from build123d import *

# Parameters (mm, degrees)
F0_W     = 60
F0_H     = 60
F1_DEPTH = 140
F2_R     = 16.4842483895
F2_R_2   = 17.1367396553
F2_R_3   = 16.9091823749
F3_DEPTH = 15
F4_DEPTH = 199
F5_DEPTH = 25
F6_DEPTH = 5


with BuildPart() as f1:
    # F0 (on Top) → F1 (new body)
    with BuildSketch(Plane.XY):
        with Locations((30, 30)):
            Rectangle(F0_W, F0_H)
    extrude(amount=F1_DEPTH)

    # F2 (on face) → F3 (join)
    with BuildSketch(Plane.XZ):
        with Locations((32.427366823, 110.1229637861)):
            Circle(F2_R)
        with Locations((32.427366823, 72.1417963505)):
            Circle(F2_R_2)
        with Locations((32.7129401267, 27.8780274093)):
            Circle(F2_R_3)
    extrude(amount=F3_DEPTH)

    # F4 (cut): a face of the model
    f4_faces = [f1.faces().sort_by_distance(p)[0] for p in [
        (32.427366823, -15, 72.1417963505),
    ]]
    extrude(f4_faces, amount=-F4_DEPTH, mode=Mode.SUBTRACT)

    # F5 (cut): a face of the model
    f5_faces = [f1.faces().sort_by_distance(p)[0] for p in [
        (32.427366823, -15, 110.1229637861),
    ]]
    extrude(f5_faces, amount=-F5_DEPTH, mode=Mode.SUBTRACT)

    # F6 (cut): a face of the model
    f6_faces = [f1.faces().sort_by_distance(p)[0] for p in [
        (32.7129401267, -15, 27.8780274093),
    ]]
    extrude(f6_faces, amount=-F6_DEPTH, mode=Mode.SUBTRACT)


solid = f1.part
Could you check a few things on this model? Use its own coordinates, in mm. A direction names the side the tool comes from. Round coordinates to 2 decimals unless told otherwise and drop trailing zeros. Order: outer loops, then holes, each group sorted by start corner. A loop starts at its lowest first (then second) coordinate and runs counter-clockwise, first axis right, second up.
(1) Imagine slicing it at D-D (z = 20). Write out the boundary of the cut face in (x, y).
Response values:
outline: (0, 0) - (17.75, 0) - (17.75, -10) - (47.67, -10) - (47.67, 0) - (60, 0) - (60, 60) - (0, 60) - close
(2) Which directions (+Z, -Z, +X, -X, +Y, -Y) give clear straight access to the entire face, cutting with the end or side of a thin tool? Please do faces 4 (the flat face through (32, -10, 28)), 5 (the flat face through (32, 10, 110)).
Response values:
face 4: +Z, -Z, +X, -X, -Y
face 5: -Y
(3) Please list where these lines run through material, in increasing order: line 1 along Z through (x, y) = (26, 6.5); line 2 along Z through (x, y) = (33, 26.5); line 3 along Z through (x, y) = (25, 7).
Response values:
line 1: z = 0 to 56.26, 88.03 to 94.94, 125.3 to 140
line 2: z = 0 to 55.01, 89.27 to 140
line 3: z = 0 to 56.7, 87.59 to 95.41, 124.84 to 140
(4) Imagine slicing it at C-C (y = 28). Write out the boundary of the cut face in (x, z).
Response values:
outline: (0, 0) - (60, 0) - (60, 140) - (0, 140) - close; hole circle Ø34.27 at (32.43, 72.14)
(5) Imagine slicing it at A-A (x = 29.5). Write out the boundary of the cut face in (y, z), plus the area to 3 significant figures.
Response values:
outline: (-10, 11.28) - (0, 11.28) - (0, 0) - (60, 0) - (60, 55.26) - (0, 55.26) - (0, 44.48) - (-10, 44.48) - close; (0, 89.03) - (60, 89.03) - (60, 140) - (0, 140) - (0, 126.35) - (10, 126.35) - (10, 93.9) - (0, 93.9) - close
area: 6,380 mm2
(6) Imagine slicing it at B-B (z = 73.5). Write out the boundary of the cut face in (x, y).
Response values:
outline: (0, 0) - (15.34, 0) - (15.34, 60) - (0, 60) - close; (49.51, 0) - (60, 0) - (60, 60) - (49.51, 60) - close
(7) I'm going to push flat-ended pins straight in: pin 1 (10 mm diameter, centred on x = 35, z = 116.5, fed in from -Y); pin 2 (18 mm diameter, centred on x = 15.5, z = 79, fed in from -Y). Where does each tip first touch, or does it pass through?
Response values:
pin 1: stops at y = 10
pin 2: stops at y = 0
(8) If we mould it in two halves opening along Z, with no side actions, what happens to faces 1 (the cylindrical face through (28.712, 29.58, 55.413)), 2 (the flat face through (0, 30, 69)), 3 (the flat face through (30, 30, 140))? For each: released by +Z, released by -Z, zero draft, split by the parting line, or undercut.
Response values:
face 1: undercut
face 2: zero draft
face 3: released by +Z
